```python
from build123d import *

# Parameters (mm, degrees)
BOSS_EXTRUDE1_DEPTH = 94.5
CUT_EXTRUDE1_DEPTH  = 1
CHAMFER3_SIZE       = 1.5
CHAMFER3_SIZE_2     = 1.050311307
SKETCH3_W           = 12.8
SKETCH3_H           = 5.35
CUT_EXTRUDE2_DEPTH  = 6
CUT_EXTRUDE3_DEPTH  = 6
CUT_EXTRUDE4_DEPTH  = 6
FILLET1_R           = 8


with BuildPart() as part:
    # Sketch1 → Boss-Extrude1 (new body)
    with BuildSketch(Plane.XY):
        with BuildLine():
            Line((19.875, 11.625), (-19.875, 11.625))
            ThreePointArc((-19.875, 11.625), (-31.5, 0), (-19.875, -11.625))
            Line((-19.875, -11.625), (19.875, -11.625))
            ThreePointArc((19.875, -11.625), (31.5, 0), (19.875, 11.625))
        make_face()
    extrude(amount=BOSS_EXTRUDE1_DEPTH)

    # Sketch2 → Cut-Extrude1 (cut)
    with BuildSketch(Plane(origin=(0, 0, 0), x_dir=(-1, 0, 0), z_dir=(0, 0, -1))):
        with BuildLine():
            Line((20.45, 6.05), (-20.45, 6.05))
            ThreePointArc((-20.45, 6.05), (-26.5, 0), (-20.45, -6.05))
            Line((-20.45, -6.05), (20.45, -6.05))
            ThreePointArc((20.45, -6.05), (26.5, 0), (20.45, 6.05))
        make_face()
    extrude(amount=-CUT_EXTRUDE1_DEPTH, mode=Mode.SUBTRACT)

    # Chamfer3
    # the kernel refuses this chamfer: 1.5, 1.050311307 mm, written as the material it takes off along each edge
    with BuildSketch(Plane(origin=(-20.45, 0, 0), x_dir=(0, -1, 0), z_dir=(1, 0, 0))) as chamfer3_piece_1_section:
        Polygon((6.05 + CHAMFER3_SIZE, 0), (6.05, -CHAMFER3_SIZE_2), (6.05, 0), align=None)
    chamfer3_piece_1 = revolve(axis=Axis((-20.45, 0, 0), (0, 0, -1)), revolution_arc=180, mode=Mode.PRIVATE)
    chamfer3_piece_1 = split(chamfer3_piece_1, bisect_by=Plane(origin=(-27.29545789, 0, 1), z_dir=(0, 0, -1)), keep=Keep.TOP, mode=Mode.PRIVATE)
    add(chamfer3_piece_1, mode=Mode.SUBTRACT)
    with BuildSketch(Plane(origin=(-20.45, 6.05, 0), x_dir=(0, 0.9997533347641299, -0.022209674198457065), z_dir=(1, 0, 0))) as chamfer3_piece_2_section:
        Polygon((CHAMFER3_SIZE * 0.999753334764, CHAMFER3_SIZE * 0.0222096741985), (-CHAMFER3_SIZE_2 * 0.0222096742051, CHAMFER3_SIZE_2 * 0.999753335064), (0, 0), align=None)
    chamfer3_piece_2 = extrude(amount=40.9, mode=Mode.PRIVATE)
    chamfer3_piece_2 = split(chamfer3_piece_2, bisect_by=Plane(origin=(0, 6.554046445, 1), z_dir=(0, 0, -1)), keep=Keep.TOP, mode=Mode.PRIVATE)
    add(chamfer3_piece_2, mode=Mode.SUBTRACT)
    with BuildSketch(Plane(origin=(20.45, -6.05, 0), x_dir=(0, -0.9997533347641299, -0.022209674198457065), z_dir=(-1, 0, 0))) as chamfer3_piece_3_section:
        Polygon((CHAMFER3_SIZE * 0.999753334764, CHAMFER3_SIZE * 0.0222096741985), (-CHAMFER3_SIZE_2 * 0.0222096742051, CHAMFER3_SIZE_2 * 0.999753335064), (0, 0), align=None)
    chamfer3_piece_3 = extrude(amount=40.9, mode=Mode.PRIVATE)
    chamfer3_piece_3 = split(chamfer3_piece_3, bisect_by=Plane(origin=(0, -6.554046445, 1), z_dir=(0, 0, -1)), keep=Keep.TOP, mode=Mode.PRIVATE)
    add(chamfer3_piece_3, mode=Mode.SUBTRACT)
    with BuildSketch(Plane(origin=(20.45, 0, 0), x_dir=(0, 1, 0), z_dir=(-1, 0, 0))) as chamfer3_piece_4_section:
        Polygon((6.05 + CHAMFER3_SIZE, 0), (6.05, -CHAMFER3_SIZE_2), (6.05, 0), align=None)
    chamfer3_piece_4 = revolve(axis=Axis((20.45, 0, 0), (0, 0, -1)), revolution_arc=180, mode=Mode.PRIVATE)
    chamfer3_piece_4 = split(chamfer3_piece_4, bisect_by=Plane(origin=(27.295457889, 0, 1), z_dir=(0, 0, -1)), keep=Keep.TOP, mode=Mode.PRIVATE)
    add(chamfer3_piece_4, mode=Mode.SUBTRACT)

    # Sketch3 → Cut-Extrude2 (cut)
    with BuildSketch(Plane(origin=(0, 0, 1), x_dir=(-1, 0, 0), z_dir=(0, 0, -1))):
        with Locations((-17.171851993, 0)):
            Rectangle(SKETCH3_W, SKETCH3_H)
        with Locations((17.171851993, 0)):
            Rectangle(SKETCH3_W, SKETCH3_H)
    extrude(amount=-CUT_EXTRUDE2_DEPTH, mode=Mode.SUBTRACT)

    # Sketch3<3> → Cut-Extrude3 (cut)
    with BuildSketch(Plane(origin=(0, 0, 1), x_dir=(-1, 0, 0), z_dir=(0, 0, -1))):
        Polygon((-3.45, -2.675), (3.45, -2.675), (3.45, -1.575), (2.7, -0.825), (-2.7, -0.825), (-3.45, -1.575), align=None)
    extrude(amount=-CUT_EXTRUDE3_DEPTH, mode=Mode.SUBTRACT)

    # Sketch3<4> → Cut-Extrude4 (cut)
    with BuildSketch(Plane(origin=(0, 0, 1), x_dir=(-1, 0, 0), z_dir=(0, 0, -1))):
        with BuildLine():
            Line((-2.85, 1.735925997), (2.85, 1.735925997))
            ThreePointArc((2.85, 1.735925997), (4.175, 3.060925997), (2.85, 4.385925997))
            Line((2.85, 4.385925997), (-2.85, 4.385925997))
            ThreePointArc((-2.85, 4.385925997), (-4.175, 3.060925997), (-2.85, 1.735925997))
        make_face()
    extrude(amount=-CUT_EXTRUDE4_DEPTH, mode=Mode.SUBTRACT)

    # Fillet1
    # the kernel refuses this fillet: 8 mm, written as the material it takes off along each edge
    with BuildSketch(Plane(origin=(19.875, 0, 0), x_dir=(0, -1, 0), z_dir=(-1, 0, 0))) as fillet1_piece_1:
        with BuildLine():
            CenterArc((11.625 - FILLET1_R, FILLET1_R), FILLET1_R, 270, 90)
            Line((11.625 - FILLET1_R, 0), (11.625, 0))
            Line((11.625, 0), (11.625, FILLET1_R))
        make_face()
    revolve(axis=Axis((19.875, 0, 0), (0, 0, 1)), revolution_arc=180, mode=Mode.SUBTRACT)
    with BuildSketch(Plane(origin=(-19.875, -11.625, 0), x_dir=(0, 0, 1), z_dir=(1, 0, 0)), Plane(origin=(19.875, 11.625, 94.5), x_dir=(0, -1, 0), z_dir=(-1, 0, 0))) as fillet1_piece_2:
        with BuildLine():
            CenterArc((FILLET1_R, -FILLET1_R), FILLET1_R, 90, 90)
            Line((0, -FILLET1_R), (0, 0))
            Line((0, 0), (FILLET1_R, 0))
        make_face()
    extrude(amount=39.75, mode=Mode.SUBTRACT)
    with BuildSketch(Plane(origin=(-19.875, 0, 0), x_dir=(0, 1, 0), z_dir=(1, 0, 0))) as fillet1_piece_3:
        with BuildLine():
            CenterArc((11.625 - FILLET1_R, FILLET1_R), FILLET1_R, 270, 90)
            Line((11.625 - FILLET1_R, 0), (11.625, 0))
            Line((11.625, 0), (11.625, FILLET1_R))
        make_face()
    revolve(axis=Axis((-19.875, 0, 0), (0, 0, 1)), revolution_arc=180, mode=Mode.SUBTRACT)
    with BuildSketch(Plane(origin=(19.875, 0, 94.5), x_dir=(0, -1, 0), z_dir=(-1, 0, 0))) as fillet1_piece_4:
        with BuildLine():
            CenterArc((11.625 - FILLET1_R, -FILLET1_R), FILLET1_R, 0, 90)
            Line((11.625 - FILLET1_R, 0), (11.625, 0))
            Line((11.625, 0), (11.625, -FILLET1_R))
        make_face()
    revolve(axis=Axis((19.875, 0, 94.5), (0, 0, 1)), revolution_arc=180, mode=Mode.SUBTRACT)
    with BuildSketch(Plane(origin=(-19.875, -11.625, 94.5), x_dir=(0, 0, -1), z_dir=(1, 0, 0)), Plane(origin=(19.875, 11.625, 0), x_dir=(0, -1, 0), z_dir=(-1, 0, 0))) as fillet1_piece_5:
        with BuildLine():
            CenterArc((FILLET1_R, FILLET1_R), FILLET1_R, 180, 90)
            Line((0, FILLET1_R), (0, 0))
            Line((0, 0), (FILLET1_R, 0))
        make_face()
    extrude(amount=39.75, mode=Mode.SUBTRACT)
    with BuildSketch(Plane(origin=(-19.875, 0, 94.5), x_dir=(0, 1, 0), z_dir=(1, 0, 0))) as fillet1_piece_6:
        with BuildLine():
            CenterArc((11.625 - FILLET1_R, -FILLET1_R), FILLET1_R, 0, 90)
            Line((11.625 - FILLET1_R, 0), (11.625, 0))
            Line((11.625, 0), (11.625, -FILLET1_R))
        make_face()
    revolve(axis=Axis((-19.875, 0, 94.5), (0, 0, 1)), revolution_arc=180, mode=Mode.SUBTRACT)


solid = part.part
```
Check sheet for the modelled part. Datum: model origin and axes. Units: mm. A direction names the side the tool comes from. Give positions to 0.01 mm unless a question says otherwise; leave off trailing zeros. Order: outer loops, then holes, each group sorted by start corner. A loop starts at its lowest first (then second) coordinate and runs counter-clockwise, first axis right, second up. Notation, with made-up numbers: (49.25, 39.25) -> (60.25, 39.25) arc R27 ccw to (60.25, 69.25) -> close; hole circle Ø9 at (-14.5, -23). An arc over 180 degrees is marked (long way). Return JSON: item names as keys, results as strings.
1. Material ranges on probe 1 along Z at (x, y) = (8, -2.75); probe 2 along Z at (x, y) = (-1.5, 2.75); probe 3 along Y at (x, z) = (-20, 11), recorded low to high. Write a range as [from, to].
From the geometry:
{"probe 1": "[1, 94.5]", "probe 2": "[7, 94.5]", "probe 3": "[-11.62, 11.62]"}
2. Mould release check, pull along X, two halves, no side actions. Record for faces 3 (the cylindrical face through (31.497, -0.256, 46.7)), 4 (the cylindrical face through (-0.278, -10.312, 3.609)), 5 (the flat face through (-10.772, 0, 4)): +X half, -X half, draft (parallel to the pull), parting line (faces both ways), or undercut.
From the geometry:
{"face 3": "+X half", "face 4": "draft", "face 5": "undercut"}
3. Set-up check for faces 1 (the cylindrical face through (0.278, 10.312, 3.609)), 2 (the flat face through (0, 4.386, 4)): record each of +Z, -Z, +X, -X, +Y, -Y from which the full face is reachable in a straight line by a thin tool's end or side.
From the geometry:
{"face 1": "-Z, +X, -X, +Y", "face 2": "-Z"}
4. Cross-section at B-B, the plane z = 15. Record the cut outline in (x, y) (3 decimals).
From the geometry:
{"outline": "(-19.875, -11.625) -> (19.875, -11.625) arc R11.625 ccw to (19.875, 11.625) -> (-19.875, 11.625) arc R11.625 ccw to start"}
5. Go/stop test with flat-tipped pins: P1, Ø5, axis at x = 18, z = 5, coming from the +Y side; P2, Ø4.5, axis at y = 0, z = 3.5, coming from the -X side; P3, Ø1.5, axis at x = 6.5, y = -1.5, coming from the -Z side. Record where each tip stops, or that it passes through.
From the geometry:
{"P1": "y = 11.61", "P2": "x = -31.18", "P3": "z = 1"}
6. Cross-section at A-A, the plane x = 16.5. Record the cut outline in (y, z) (3 decimals).
From the geometry:
{"outline": "(-11.625, 8) arc R8 ccw to (-6.683, 0.607) -> (-6.122, 1) -> (-2.675, 1) -> (-2.675, 7) -> (2.675, 7) -> (2.675, 1) -> (6.122, 1) -> (6.683, 0.607) arc R8 ccw to (11.625, 8) -> (11.625, 86.5) arc R8 ccw to (3.625, 94.5) -> (-3.625, 94.5) arc R8 ccw to (-11.625, 86.5) -> close"}
